Model file for the job. Use its own axes, mm. A direction names the side the tool comes from. Coordinates: 2 decimals unless noted, no trailing zeros. Write each loop counter-clockwise with the first axis right and the second up, starting at its lowest first coordinate (ties: lowest second). Pieces come first, ordered by that corner, then holes. Notation, with made-up numbers: (70, -3) - (126, -3) arc R8 cw to (126, 4) - close; hole circle Ø5 at (0.5, 84.5). An arc over 180 degrees is marked (long way). Put each result on its own line as item: value. Start each with the question number.
1. Saw through at A-A, the plane z = 1.5. Write the cut outline in (x, y), plus the area to 3 significant figures.
2. Which spindle directions (+Z, -Z, +X, -X, +Y, -Y) get a long thin tool onto all of the face, cutting with end or side? Do faces 4 (the face through (-287.222, -12.641, 12.43)), 5 (the face through (-287.222, -12.641, -12.57)), 6 (the face through (4, 0, 17.5)). Say none if no direction does.
3. Pull direction X, two halves, no side cores. Call faces 1 (the face through (-5.937, 26.734, -16.874)), 2 (the face through (-40.68, -309.84, 0.11)), 3 (the face through (-267, 111, -17.5)): released by +X, released by -X, zero draft, split by the parting line, or undercut.
4. Drop flat-ended pins along their axis: P1, Ø2, axis at y = -248, z = 10.5, coming from the -X side; P2, Ø12, axis at y = 175.5, z = 6.5, coming from the +X side; P3, Ø10, axis at x = -61, y = -53.5, coming from the +Z side. Give the stop position or say it passes through.
5. Drill centre lines: L1, parallel to Y at x = 0, z = 1; L2, parallel to Z at x = -213.5, y = -34.5; L3, parallel to Y at x = 112, z = -14. Where is each one in solid material? Low to high. Write a range as from..to.
```python
from build123d import *

# Parameters (mm, degrees)
SKETCH5_R          = 3.75
CUT_EXTRUDE1_DEPTH = 72


with BuildPart() as part:
    # Sketch3 → Revolve2 (revolve)
    with BuildSketch(Plane(origin=(0, 0, 0), x_dir=(1, 0, 0), z_dir=(0, 1, 0))):
        with BuildLine():
            Line((287.5, 17.5), (302.5, 17.5))
            ThreePointArc((302.5, 17.5), (309.571067812, 14.571067812), (312.5, 7.5))
            Line((312.5, 7.5), (312.5, -7.5))
            ThreePointArc((312.5, -7.5), (309.571067812, -14.571067812), (302.5, -17.5))
            Line((302.5, -17.5), (287.5, -17.5))
            Line((287.5, -17.5), (287.5, -7.5))
            Line((287.5, -7.5), (10.028182078, -17.5))
            Line((10.028182078, -17.5), (0, -17.5))
            Line((0, -17.5), (0, 17.5))
            Line((0, 17.5), (10.028182078, 17.5))
            Line((10.028182078, 17.5), (287.5, 7.5))
            Line((287.5, 7.5), (287.5, 17.5))
        make_face()
    revolve(axis=Axis((0, 0, 17.5), (0, 0, -1)))

    # Sketch5 → Cut-Extrude1 (cut)
    with BuildSketch(Plane.XY.offset(17.5)):
        Circle(SKETCH5_R)
    extrude(amount=-CUT_EXTRUDE1_DEPTH, mode=Mode.SUBTRACT)


solid = part.part
```
Final values:
1. outline: circle Ø625 at (0, 0); hole circle Ø7.5 at (0, 0)
1. area: 307,000 mm²
2. face 4: +Z
2. face 5: -Z
2. face 6: +Z, +X, -X, +Y, -Y
3. face 1: undercut
3. face 2: split by the parting line
3. face 3: zero draft
4. P1: stops at x = -190.77
4. P2: stops at x = 262.54
4. P3: stops at z = 15.12
5. L1: y = -312.5..-3.75, 3.75..312.5
5. L2: z = -10.07..10.07
5. L3: y = -289.17..-264.79, 264.79..289.17
